Verification items for the finished model (mm, model axes). Round coordinates to 2 decimals unless told otherwise and drop trailing zeros. Loops run counter-clockwise (first coordinate to the right, second up) from the corner with the lowest first, then second, coordinate; pieces in that order, holes last. Notation, with made-up numbers: (-12, -30.75) -> (14, -30.75) arc R14 ccw to (14, -11.75) -> close; hole circle Ø9 at (-7.75, -15). An arc over 180 degrees is marked (long way). Use a Markdown table: item, result. Add a question column.
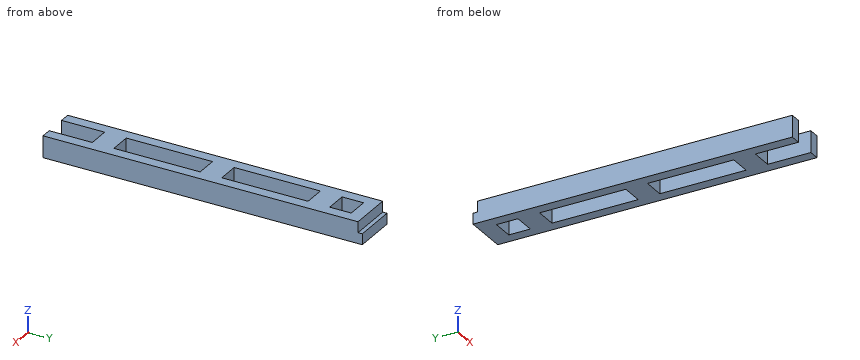
```python
from build123d import *

# Parameters (mm, degrees)
F0_W     = 10
F0_H     = 10
F1_DEPTH = 10
F2_W     = 10
F2_H     = 10
F3_DEPTH = 10
F4_W     = 20
F4_H     = 8
F5_DEPTH = 5
F6_W     = 20
F6_H     = 6
F7_DEPTH = 5


with BuildPart() as f1:
    # F0 (on Top) → F1 (new body)
    with BuildSketch(Plane.XY):
        Polygon((0, 140), (0, 0), (5, 0), (5, 20), (5, 30), (5, 70), (5, 80), (5, 120), (5, 130), (5, 140), align=None)
        with Locations((10, 25)):
            Rectangle(F0_W, F0_H)
        Polygon((15, 30), (15, 20), (15, 0), (20, 0), (20, 140), (15, 140), (15, 130), (15, 120), (15, 80), (15, 70), align=None)
        with Locations((10, 125)):
            Rectangle(F0_W, F0_H)
    extrude(amount=F1_DEPTH)

    # F2 (on Top) → F3 (join)
    with BuildSketch(Plane.XY):
        with Locations((10, 75)):
            Rectangle(F2_W, F2_H)
    extrude(amount=F3_DEPTH)

    # F4 (on Top) → F5 (join)
    with BuildSketch(Plane.XY):
        with Locations((10, 144)):
            Rectangle(F4_W, F4_H)
    extrude(amount=F5_DEPTH)

    # F6 (on face) → F7 (join)
    with BuildSketch(Plane.XY.offset(5)):
        with Locations((10, 143)):
            Rectangle(F6_W, F6_H)
    extrude(amount=F7_DEPTH)


solid = f1.part
```
1) Sectioned sample at C-C on z = 7.5. Enter the section's corners in (x, y), then the cut area to 3 significant figures.
2) Go/stop test with flat-tipped pins: pin 1 (3 mm diameter, centred on x = 8.5, z = 3, fed in from -Y); pin 2 (5 mm diameter, centred on x = 17, z = 7, fed in from +Y); pin 3 (2.5 mm diameter, centred on x = 10.5, z = 6.5, fed in from +Y). Record where each tip stops, or that it passes through.
3) Sectioned sample at B-B on x = 7.5. Enter the section's corners in (y, z), then the cut area to 3 significant figures.
4) Thickness scan on line 1 (Y direction, x = 9.75, z = 7); line 2 (Y direction, x = 7, z = 1.5); line 3 (X direction, y = 46.5, z = 3.25). Record the ranges inside material, lowest first.
5) Sectioned sample at A-A on y = 95.5. Enter the section's corners in (x, z), then the cut area to 3 significant figures.
Geometry results:
| question | item | result |
|---|---|---|
| 1 | outline | (0, 0) -> (5, 0) -> (5, 20) -> (15, 20) -> (15, 0) -> (20, 0) -> (20, 146) -> (0, 146) -> close; hole (5, 30) -> (15, 30) -> (15, 70) -> (5, 70) -> close; hole (5, 80) -> (15, 80) -> (15, 120) -> (5, 120) -> close; hole (5, 130) -> (15, 130) -> (15, 140) -> (5, 140) -> close |
| 1 | area | 1,820 mm^2 |
| 2 | pin 1 | y = 20 |
| 2 | pin 2 | y = 148 |
| 2 | pin 3 | y = 146 |
| 3 | outline | (20, 0) -> (30, 0) -> (30, 10) -> (20, 10) -> close; (70, 0) -> (80, 0) -> (80, 10) -> (70, 10) -> close; (120, 0) -> (130, 0) -> (130, 10) -> (120, 10) -> close; (140, 0) -> (148, 0) -> (148, 5) -> (146, 5) -> (146, 10) -> (140, 10) -> close |
| 3 | area | 370 mm^2 |
| 4 | line 1 | 20 to 30, 70 to 80, 120 to 130, 140 to 146 |
| 4 | line 2 | 20 to 30, 70 to 80, 120 to 130, 140 to 148 |
| 4 | line 3 | 0 to 5, 15 to 20 |
| 5 | outline | (0, 0) -> (5, 0) -> (5, 10) -> (0, 10) -> close; (15, 0) -> (20, 0) -> (20, 10) -> (15, 10) -> close |
| 5 | area | 100 mm^2 |
